```python
from build123d import *

# Parameters (mm, degrees)
SKETCH_1_R      = 2
EXTRUDE_1_DEPTH = 6


with BuildPart() as part:
    # Эскиз1 → Бобышка-Вытянуть1 (new body)
    with BuildSketch(Plane.XY):
        with BuildLine():
            Line((-16, -50), (16, -50))
            ThreePointArc((16, -50), (19.535533906, -48.535533906), (21, -45))
            Line((21, -45), (21, -12.071067812))
            ThreePointArc((21, -12.071067812), (24.086582838, -7.451670149), (29.535533906, -8.535533906))
            Line((29.535533906, -8.535533906), (51.405591591, -30.405591591))
            ThreePointArc((51.405591591, -30.405591591), (54.941125497, -31.870057685), (58.476659403, -30.405591591))
            Line((58.476659403, -30.405591591), (81.104076401, -7.778174593))
            ThreePointArc((81.104076401, -7.778174593), (82.568542495, -4.242640687), (81.104076401, -0.707106781))
            Line((81.104076401, -0.707106781), (22.464466094, 57.932503526))
            ThreePointArc((22.464466094, 57.932503526), (20.84234935, 59.016367282), (18.928932188, 59.39696962))
            Line((18.928932188, 59.39696962), (-18.928932188, 59.39696962))
            ThreePointArc((-18.928932188, 59.39696962), (-20.84234935, 59.016367282), (-22.464466094, 57.932503526))
            Line((-22.464466094, 57.932503526), (-81.104076401, -0.707106781))
            ThreePointArc((-81.104076401, -0.707106781), (-82.568542495, -4.242640687), (-81.104076401, -7.778174593))
            Line((-81.104076401, -7.778174593), (-58.476659403, -30.405591591))
            ThreePointArc((-58.476659403, -30.405591591), (-54.941125497, -31.870057685), (-51.405591591, -30.405591591))
            Line((-51.405591591, -30.405591591), (-29.535533906, -8.535533906))
            ThreePointArc((-29.535533906, -8.535533906), (-24.086582838, -7.451670149), (-21, -12.071067812))
            Line((-21, -12.071067812), (-21, -45))
            ThreePointArc((-21, -45), (-19.535533906, -48.535533906), (-16, -50))
        make_face()
        with Locations((-70.497474683, -4.242640687)):
            Circle(SKETCH_1_R, mode=Mode.SUBTRACT)
        with Locations((-54.941125497, -19.798989873)):
            Circle(SKETCH_1_R, mode=Mode.SUBTRACT)
        with Locations((-42.213203436, 24.04163056)):
            Circle(SKETCH_1_R, mode=Mode.SUBTRACT)
        with Locations((-26.656854249, 8.485281374)):
            Circle(SKETCH_1_R, mode=Mode.SUBTRACT)
        with Locations((-11, -40)):
            Circle(SKETCH_1_R, mode=Mode.SUBTRACT)
        with Locations((-11, 49.39696962)):
            Circle(SKETCH_1_R, mode=Mode.SUBTRACT)
        with Locations((-11, -4.242640687)):
            Circle(SKETCH_1_R, mode=Mode.SUBTRACT)
        with Locations(Location((11, -40, 0), (0, 0, 180))):
            Circle(SKETCH_1_R, mode=Mode.SUBTRACT)
        with Locations(Location((11, -4.242640687, 0), (0, 0, 180))):
            Circle(SKETCH_1_R, mode=Mode.SUBTRACT)
        with Locations(Location((26.656854249, 8.485281374, 0), (0, 0, 180))):
            Circle(SKETCH_1_R, mode=Mode.SUBTRACT)
        with Locations(Location((54.941125497, -19.798989873, 0), (0, 0, 180))):
            Circle(SKETCH_1_R, mode=Mode.SUBTRACT)
        with Locations(Location((70.497474683, -4.242640687, 0), (0, 0, 180))):
            Circle(SKETCH_1_R, mode=Mode.SUBTRACT)
        with Locations(Location((42.213203436, 24.04163056, 0), (0, 0, 180))):
            Circle(SKETCH_1_R, mode=Mode.SUBTRACT)
        with Locations(Location((11, 49.39696962, 0), (0, 0, 180))):
            Circle(SKETCH_1_R, mode=Mode.SUBTRACT)
    extrude(amount=EXTRUDE_1_DEPTH)


solid = part.part
```
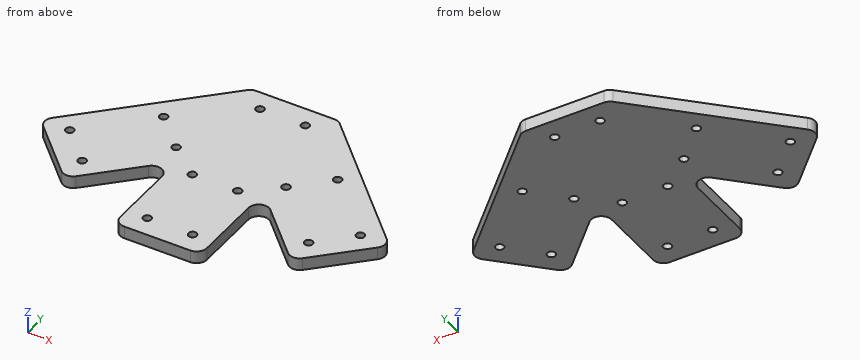
Part model, mm, in its own coordinate system. Give positions to 0.01 mm unless a question says otherwise; leave off trailing zeros. Order: outer loops, then holes, each group sorted by start corner. A loop starts at its lowest first (then second) coordinate and runs counter-clockwise, first axis right, second up. Notation, with made-up numbers: (20.25, -29) - (31.25, -29) arc R15 cw to (31.25, -3) - close; hole circle Ø3 at (70, 21). An arc over 180 degrees is marked (long way). Use one line per item in the form item = value.
Item 1: Pin check, flat tip, straight feed: pin 1 Ø1.8 at (y, z) = (-27, 2.5) entering from -X. Stop position of the tip, or through.
Solution:
pin_1 = -62.78
Item 2: Slice it at B-B on y = -40. Give the cut face in (x, z), and give its area (3 significant figures).
Solution:
outline = (-21, 0) - (-13, 0) - (-13, 6) - (-21, 6) - close; (-9, 0) - (9, 0) - (9, 6) - (-9, 6) - close; (13, 0) - (21, 0) - (21, 6) - (13, 6) - close
area = 204 mm2
Item 3: Slice it at A-A on x = -11. Give the cut face in (y, z).
Solution:
outline = (-50, 0) - (-42, 0) - (-42, 6) - (-50, 6) - close; (-38, 0) - (-6.24, 0) - (-6.24, 6) - (-38, 6) - close; (-2.24, 0) - (47.4, 0) - (47.4, 6) - (-2.24, 6) - close; (51.4, 0) - (59.4, 0) - (59.4, 6) - (51.4, 6) - close
Item 4: Slice it at D-D on z = 1.5. Count the separate pieces of the cut face and the enclosed holes in it, and give its area (3 significant figures).
Solution:
separate_pieces = 1
enclosed_holes = 14
area = 10,200 mm2
Item 5: Probe probe 1 along Y at (x, z) = (11, 2.15); probe 2 along X at (y, z) = (-31, 2); probe 3 along X at (y, z) = (-11.5, 2.85). List the from-to ranges inside material, lowest first. Write a range as from..to.
Solution:
probe_1 = -50..-42, -38..-6.24, -2.24..47.4, 51.4..59.4
probe_2 = -57.76..-52.12, -21..21, 52.12..57.76
probe_3 = -77.38..-32.5, -21.03..21.03, 32.5..77.38
Item 6: Slice it at C-C on x = -55. Give the cut face in (y, z).
Solution:
outline = (-31.87, 0) - (-21.8, 0) - (-21.8, 6) - (-31.87, 6) - close; (-17.8, 0) - (25.4, 0) - (25.4, 6) - (-17.8, 6) - close
